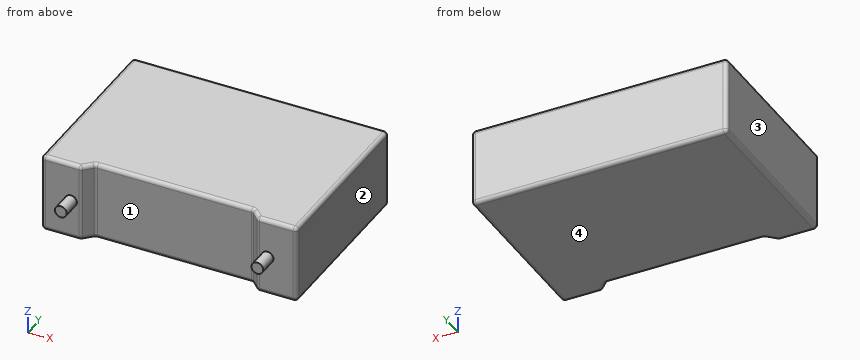
```python
from build123d import *

# Parameters (mm, degrees)
SKETCH1_W           = 13
SKETCH1_H           = 4
BOSS_EXTRUDE1_DEPTH = 9
CUT_EXTRUDE1_DEPTH  = 5
SKETCH3_R           = 0.3
BOSS_EXTRUDE2_DEPTH = 1
FILLET1_R           = 0.2


with BuildPart() as part:
    # Sketch1 → Boss-Extrude1 (new body)
    with BuildSketch(Plane(origin=(0, 0, 0), x_dir=(1, 0, 0), z_dir=(0, 1, 0))):
        Rectangle(SKETCH1_W, SKETCH1_H)
    extrude(amount=BOSS_EXTRUDE1_DEPTH)

    # Sketch2 → Cut-Extrude1 (cut, through all)
    with BuildSketch(Plane.XY.offset(2)):
        Polygon((-4.5, 0), (-4, 0.5), (4, 0.5), (4.5, 0), (4.5, -1.5), (-4.5, -1.5), align=None)
    extrude(amount=-CUT_EXTRUDE1_DEPTH, mode=Mode.SUBTRACT)

    # Sketch3 → Boss-Extrude2 (add)
    with BuildSketch(Plane.XZ):
        with Locations((5, 0)):
            Circle(SKETCH3_R)
        with Locations((-5, 0)):
            Circle(SKETCH3_R)
    extrude(amount=BOSS_EXTRUDE2_DEPTH)

    # Fillet1
    fillet1_edges = [part.edges().sort_by_distance(p)[0] for p in [
        (6.5, 9, 0),
        (0, 9, -2),
        (-5.5, 0, -2),
        (5.5, 0, 2),
        (4.25, 0.25, 2),
        (0, 0.5, 2),
        (-4.25, 0.25, 2),
        (-4.25, 0.25, -2),
        (-4.5, 0, 0),
        (0, 0.5, -2),
        (-4, 0.5, 0),
        (4.25, 0.25, -2),
        (4, 0.5, 0),
        (4.5, 0, 0),
        (-6.5, 9, 0),
        (5.5, 0, -2),
        (6.5, 0, 0),
        (-5.5, 0, 2),
        (-6.5, 0, 0),
        (0, 9, 2),
        (-6.5, 4.5, -2),
        (6.5, 4.5, -2),
        (6.5, 4.5, 2),
        (-6.5, 4.5, 2),
    ]]
    fillet(fillet1_edges, radius=FILLET1_R)


solid = part.part
```
For this review, take the finished solid that the model builds, in its own axes (mm). Face numbers are marked on the shaded views. Coordinates: 2 decimals unless noted, no trailing zeros. Order: outer loops, then holes, each group sorted by start corner. A loop starts at its lowest first (then second) coordinate and runs counter-clockwise, first axis right, second up. Notation, with made-up numbers: (61.5, 58.25) -> (69.5, 58.25) arc R15 cw to (69.5, 62.25) -> close; hole circle Ø1 at (19, -20). An arc over 180 degrees is marked (long way). Answer as CSV lines item,"result".
Q1. We need section B-B (x = -0.25). State the section outline as (y, z) points.
Model answer:
outline,"(0.5, -1.8) arc R0.2 ccw to (0.7, -2) -> (8.8, -2) arc R0.2 ccw to (9, -1.8) -> (9, 1.8) arc R0.2 ccw to (8.8, 2) -> (0.7, 2) arc R0.2 ccw to (0.5, 1.8) -> close"
Q2. We need section A-A (z = 1.5). State the section outline as (x, y) points.
Model answer:
outline,"(-6.5, 0.2) arc R0.2 ccw to (-6.3, 0) -> (-4.58, 0) arc R0.2 ccw to (-4.44, 0.06) -> (-4.06, 0.44) arc R0.2 cw to (-3.92, 0.5) -> (3.92, 0.5) arc R0.2 cw to (4.06, 0.44) -> (4.44, 0.06) arc R0.2 ccw to (4.58, 0) -> (6.3, 0) arc R0.2 ccw to (6.5, 0.2) -> (6.5, 8.8) arc R0.2 ccw to (6.3, 9) -> (-6.3, 9) arc R0.2 ccw to (-6.5, 8.8) -> close"
Q3. Wall thickness on line 1 along Y through (x, z) = (2, -1.25); line 2 along Z through (x, y) = (-4.5, 0.25); line 3 along X through (y, z) = (0.25, 1.2): over which ranges is each line inside the solid? List them lowest first. Write a range as [from, to].
Model answer:
line 1,"y = [0.5, 9]"
line 2,"z = [-2, 2]"
line 3,"x = [-6.5, -4.25], [4.25, 6.5]"
Q4. We need section D-D (z = 0). State the section outline as (x, y) points, plus the area to 3 significant figures.
Model answer:
outline,"(-6.5, 0.2) arc R0.2 ccw to (-6.3, 0) -> (-5.3, 0) -> (-5.3, -1) -> (-4.7, -1) -> (-4.7, 0) -> (-4.58, 0) arc R0.2 ccw to (-4.44, 0.06) -> (-4.06, 0.44) arc R0.2 cw to (-3.92, 0.5) -> (3.92, 0.5) arc R0.2 cw to (4.06, 0.44) -> (4.44, 0.06) arc R0.2 ccw to (4.58, 0) -> (4.7, 0) -> (4.7, -1) -> (5.3, -1) -> (5.3, 0) -> (6.3, 0) arc R0.2 ccw to (6.5, 0.2) -> (6.5, 8.8) arc R0.2 ccw to (6.3, 9) -> (-6.3, 9) arc R0.2 ccw to (-6.5, 8.8) -> close"
area,"114 mm2"
Q5. We need section C-C (x = -5.5). State the section outline as (y, z) points.
Model answer:
outline,"(0, -1.8) arc R0.2 ccw to (0.2, -2) -> (8.8, -2) arc R0.2 ccw to (9, -1.8) -> (9, 1.8) arc R0.2 ccw to (8.8, 2) -> (0.2, 2) arc R0.2 ccw to (0, 1.8) -> close"
Q6. Draft analysis for pull direction X (two halves, no side actions). For the marked faces 1, 2, 3 and 4, state which applies: released by +X, released by -X, zero draft, split by the parting line, or undercut.
Model answer:
face 1,"undercut"
face 2,"released by +X"
face 3,"released by -X"
face 4,"zero draft"
Q7. Clearance check with flat-ended pins moving along their axes: pin 1 Ø1.1 at (x, z) = (0.5, 0.5) entering from -Y; pin 2 Ø1.9 at (x, z) = (6, -0.5) entering from -Y; pin 3 Ø0.5 at (x, z) = (-5.5, 0.5) entering from -Y. State where each tip first meets the part, or that it passes through.
Model answer:
pin 1,"stops at y = 0.5"
pin 2,"stops at y = -1"
pin 3,"stops at y = 0"
